Verification items for this drawing (mm, ordinates from the low corner). Round coordinates to 2 decimals unless told otherwise and drop trailing zeros. Write each loop counter-clockwise with the first axis right and the second up, starting at its lowest first coordinate (ties: lowest second). Pieces come first, ordered by that corner, then holes.
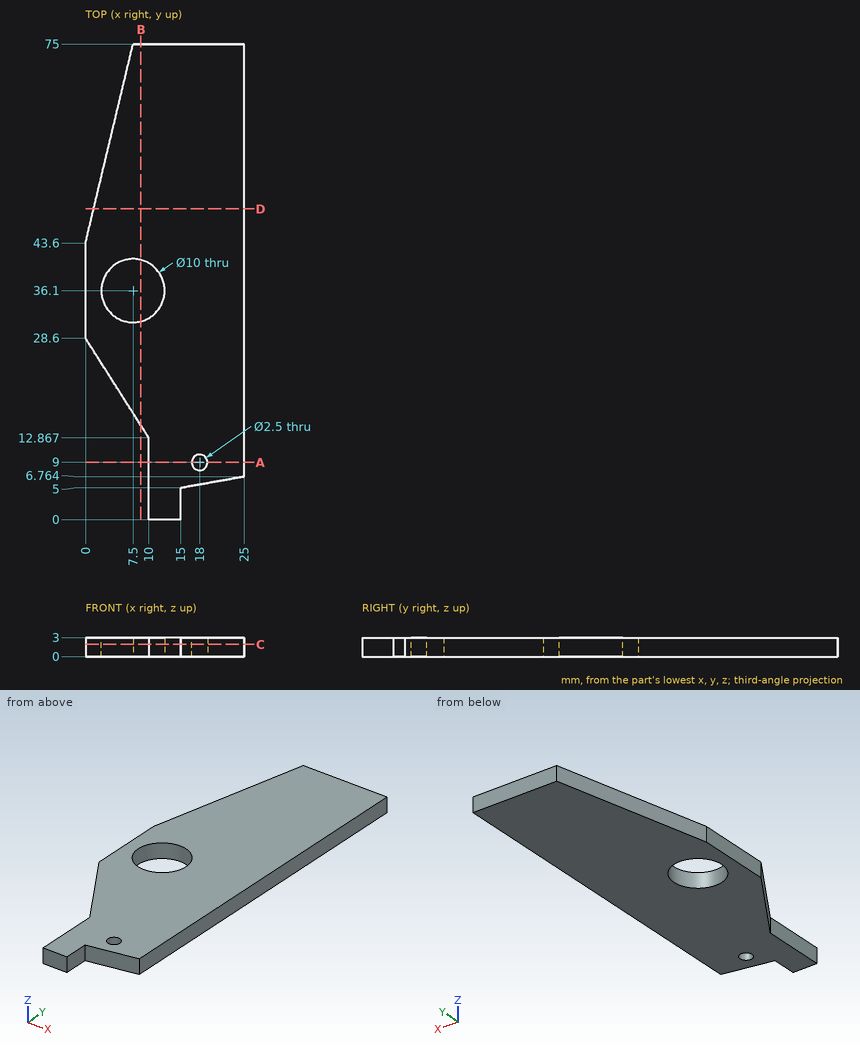
1. Scan lines: line 1 along Y through (x, z) = (8.75, 0.2) (1 decimal); line 2 along Y through (x, z) = (18, 0.7); line 3 along X through (y, z) = (62, 1.45) (1 decimal). Record each from-to range of solid material in increasing order.
2. Depth check by flat-ended pin: pin 1 Ø8 at (x, y) = (7.5, 36.1) entering from -Z; pin 2 Ø0.9 at (y, z) = (9.5, 1) entering from -X. Enter the tip coordinate at first touch or a pass-through.
3. Section check B-B (x = 8.75). Record the cut outline in (y, z).
4. Section check A-A (y = 9). Record the cut outline in (x, z).
5. Section check C-C (z = 1.9). Record the cut outline in (x, y).
6. Section check D-D (y = 49). Record the cut outline in (x, z).
Results below:
1. line 1: y = 14.8 to 31.3, 40.9 to 75
1. line 2: y = 5.53 to 7.75, 10.25 to 75
1. line 3: x = 4.4 to 25
2. pin 1: passes through
2. pin 2: stops at x = 10
3. outline: (14.83, 0) - (31.26, 0) - (31.26, 3) - (14.83, 3) - close; (40.94, 0) - (75, 0) - (75, 3) - (40.94, 3) - close
4. outline: (10, 0) - (16.75, 0) - (16.75, 3) - (10, 3) - close; (19.25, 0) - (25, 0) - (25, 3) - (19.25, 3) - close
5. outline: (0, 28.6) - (10, 12.87) - (10, 0) - (15, 0) - (15, 5) - (25, 6.76) - (25, 75) - (7.5, 75) - (0, 43.6) - close; hole circle Ø10 at (7.5, 36.1); hole circle Ø2.5 at (18, 9)
6. outline: (1.29, 0) - (25, 0) - (25, 3) - (1.29, 3) - close
